Design review of the part built by this model. Coordinates are the model's own, in mm. A direction names the side the tool comes from. Give positions to 0.01 mm unless a question says otherwise; leave off trailing zeros. Loops run counter-clockwise (first coordinate to the right, second up) from the corner with the lowest first, then second, coordinate; pieces in that order, holes last. Notation, with made-up numbers: (-34.5, 58.5) - (-22.5, 58.5) arc R29 cw to (-22.5, 78.5) - close; hole circle Ø6 at (-24.5, 71.25). An arc over 180 degrees is marked (long way). Write each question's results on one line, items separated by ' | '.
from build123d import *

# Parameters (mm, degrees)
BOSS_EXTRUDE1_DEPTH        = 2.5
F_10_0_10_DIAMETER_HOLE1_D = 10


with BuildPart() as part:
    # Sketch4 → Boss-Extrude1 (new, symmetric)
    with BuildSketch(Plane.XY):
        with BuildLine():
            Line((25, -6.698729811), (60, -6.698729811))
            Line((60, -6.698729811), (60, -24.011944979))
            Line((60, -24.011944979), (62.499998309, -25))
            Line((62.499998309, -25), (60, -30))
            Line((60, -30), (60, -70))
            Line((60, -70), (75.99999851, -70))
            Line((75.99999851, -70), (75.99999851, 62))
            Line((75.99999851, 62), (75.99999851, 65))
            Line((75.99999851, 65), (59.99999851, 65))
            Line((59.99999851, 65), (59.99999851, 62))
            Line((59.99999851, 62), (59.99999851, 57))
            ThreePointArc((59.99999851, 57), (48.111700718, 28.544206232), (19.513388562, 17.002959975))
            ThreePointArc((19.513388562, 17.002959975), (25.21513365, 5.836952637), (25, -6.698729811))
        make_face()
    extrude(amount=BOSS_EXTRUDE1_DEPTH, both=True)

    # Ø10.0 (10) Diameter Hole1 (through all)
    with Locations(Plane.XY.offset(2.5)):
        with Locations((67.99999851, 50), (67.99999851, -55)):
            Hole(F_10_0_10_DIAMETER_HOLE1_D / 2)


solid = part.part
(1) Tool access review of faces 1 (the flat face through (42, -6.699, 0)), 2 (the flat face through (61.27, -27.46, 0.04)), 3 (the flat face through (60, 61, 0)): name each direction out of +Z, -Z, +X, -X, +Y, -Y from which nothing blocks a thin tool from reaching the whole face with its end or side.
Answers below:
face 1: +Z, -Z, -X, -Y | face 2: +Z, -Z, -X | face 3: +Z, -Z, -X, +Y
(2) Take a section at A-A on y = -55. Give the boundary of the cut face in (x, z).
Answers below:
outline: (60, -2.5) - (63, -2.5) - (63, 2.5) - (60, 2.5) - close; (73, -2.5) - (76, -2.5) - (76, 2.5) - (73, 2.5) - close
(3) Take a section at B-B on z = 1.7. Give the boundary of the cut face in (x, y).
Answers below:
outline: (19.51, 17) arc R25.88 cw to (25, -6.7) - (60, -6.7) - (60, -24.01) - (62.5, -25) - (60, -30) - (60, -70) - (76, -70) - (76, 65) - (60, 65) - (60, 57) arc R40 cw to start; hole circle Ø10 at (68, -55); hole circle Ø10 at (68, 50)
(4) Take a section at D-D on y = 50. Give the boundary of the cut face in (x, z), plus the area to 3 significant figures.
Answers below:
outline: (59.38, -2.5) - (63, -2.5) - (63, 2.5) - (59.38, 2.5) - close; (73, -2.5) - (76, -2.5) - (76, 2.5) - (73, 2.5) - close | area: 33.1 mm2
(5) Take a section at C-C on x = 44.5. Give the boundary of the cut face in (y, z).
Answers below:
outline: (-6.7, -2.5) - (25.38, -2.5) - (25.38, 2.5) - (-6.7, 2.5) - close
(6) Insertion check: P1, Ø16, axis at x = 68, y = 50, coming from the -Z side; P2, Ø9, axis at x = 68, y = -55, coming from the +Z side; P3, Ø2.5, axis at y = -12, z = 1, coming from the -X side; P4, Ø1, axis at x = 54.5, z = 0, coming from the -Y side. Each pin has a flat end and moves straight along its axis. Give the tip position at first contact, or say it passes through.
Answers below:
P1: z = -2.5 | P2: through | P3: x = 60 | P4: y = -6.7
(7) Draft analysis for pull direction X (two halves, no side actions). For faces 4 (the flat face through (60, -50, 0)), 5 (the flat face through (76, -3, 0)), 6 (the cylindrical face through (73, -55, 0)), state which applies: pulls with the +X half, pulls with the -X half, needs draft (parallel to the pull), parting line crosses it, or undercut.
Answers below:
face 4: pulls with the -X half | face 5: pulls with the +X half | face 6: undercut
(8) Wall thickness on line 1 along Y through (x, z) = (67.5, 1.4); line 2 along Y through (x, z) = (67, -0.5); line 3 along Y through (x, z) = (44, 0.1): over which ranges is each line inside the solid? List them lowest first. Write a range as from..to.
Answers below:
line 1: -70..-59.97, -50.03..45.03, 54.97..65 | line 2: -70..-59.9, -50.1..45.1, 54.9..65 | line 3: -6.7..25
